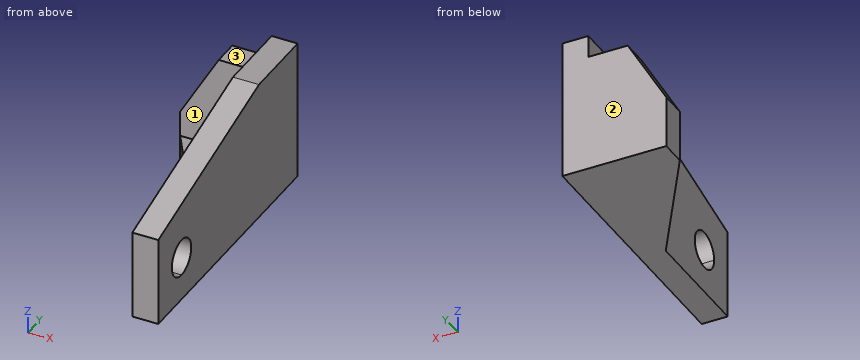
```python
from build123d import *

# Parameters (mm, degrees)
F0_W     = 33.3375
F0_H     = 11.1125
F0_W_2   = 11.1125
F1_DEPTH = 11.1125
F2_W     = 11.1125
F2_H     = 60.325
F3_DEPTH = 103.1875
F6_DEPTH = 25.4
F5_W     = 52.3875
F5_H     = 11.2454069465
F7_DEPTH = 33.3375
F9_DEPTH = 25.4


with BuildPart() as f1:
    # F0 (on Front) → F1 (new body)
    with BuildSketch(Plane.XZ):
        Polygon((-49.5353981066, -0.1329069465), (-16.1978981066, -0.1329069465), (-16.1978981066, 39.5545930535), (-33.0376141645, 39.5545930535), (-49.5353981066, 10.9795930535), align=None)
        with Locations((-32.8666481066, -5.6891569465)):
            Rectangle(F0_W, F0_H)
        with Locations((-10.6416481066, -5.6891569465)):
            Rectangle(F0_W_2, F0_H)
        Polygon((-16.1978981066, -0.1329069465), (-5.0853981066, -0.1329069465), (-5.0853981066, 49.0795930535), (-16.1978981066, 49.0795930535), (-16.1978981066, 39.5545930535), align=None)
    extrude(amount=F1_DEPTH)

    # F2 (on face) → F3 (join)
    with BuildSketch(Plane.XZ.offset(11.1125)):
        with Locations((-10.6416481066, 18.9170930535)):
            Rectangle(F2_W, F2_H)
    extrude(amount=F3_DEPTH)

    # F4 (on face) → F6 (cut)
    with BuildSketch(Plane(origin=(-16.1978981066, 0, 0), x_dir=(0, -1, 0), z_dir=(-1, 0, 0))):
        Polygon((114.3, 49.0795930535), (31.75, 49.0795930535), (114.3, 26.9603872183), align=None)
        with BuildLine():
            ThreePointArc((103.1875, 7.8045930535), (89.6373399243, 13.4172531291), (95.25, -0.1329069465))
            ThreePointArc((95.25, -0.1329069465), (100.8626600757, 2.1919329778), (103.1875, 7.8045930535))
        make_face()
    extrude(amount=-F6_DEPTH, mode=Mode.SUBTRACT)

    # F5 (on face) → F7 (join)
    with BuildSketch(Plane(origin=(-16.1978981066, 0, 0), x_dir=(0, -1, 0), z_dir=(-1, 0, 0))):
        with Locations((37.30625, -5.6227034733)):
            Rectangle(F5_W, F5_H)
    extrude(amount=F7_DEPTH)

    # F8 (on face) → F9 (cut)
    with BuildSketch(Plane.XY):
        Polygon((-16.1978981066, -63.5), (-49.5353981066, -11.1125), (-49.5353981066, -63.5), align=None)
    extrude(amount=-F9_DEPTH, mode=Mode.SUBTRACT)


solid = f1.part
```
Work out the finished part from the listing and answer in its coordinate system (mm). Face numbers are marked on the shaded views. A direction names the side the tool comes from. Give positions to 0.01 mm unless a question says otherwise; leave off trailing zeros. Order: outer loops, then holes, each group sorted by start corner. A loop starts at its lowest first (then second) coordinate and runs counter-clockwise, first axis right, second up.
1. Straight lines are drawn through the part: L1, parallel to Z at x = -27, y = -12; L2, parallel to X at y = -32, z = 11.5; L3, parallel to Y at x = -18.5, z = 32.5. For each, find the intervals that lie inside material, in ascending order.
Result sheet:
L1: z = -11.25 to 0
L2: x = -16.2 to -5.09
L3: y = -11.11 to 0
2. Section B-B, the plane y = -92.5 is taken. Determine the outline of the cut face in (x, z), and give its area (3 significant figures).
Result sheet:
outline: (-16.2, -11.25) - (-5.09, -11.25) - (-5.09, 0.36) - (-16.2, 0.36) - close; (-16.2, 15.25) - (-5.09, 15.25) - (-5.09, 32.8) - (-16.2, 32.8) - close
area: 324 mm2
3. For the marked faces 1, 2 and 3, determine the directions among +Z, -Z, +X, -X, +Y, -Y from which every point of the face is accessible in a straight line to the end or side of a thin tool.
Result sheet:
face 1: +Z, -X, -Y
face 2: +Z, -Z, +X, -X, +Y
face 3: +Z, -X, +Y, -Y
4. Section D-D, the plane y = -24 is taken. Determine the outline of the cut face in (x, z), and give its area (3 significant figures).
Result sheet:
outline: (-41.33, -11.25) - (-5.09, -11.25) - (-5.09, 49.08) - (-16.2, 49.08) - (-16.2, 0) - (-41.33, 0) - close
area: 953 mm2
5. Section C-C, the plane z = 36 is taken. Determine the outline of the cut face in (x, y), and give its area (3 significant figures).
Result sheet:
outline: (-35.09, -11.11) - (-16.2, -11.11) - (-16.2, -80.56) - (-5.09, -80.56) - (-5.09, 0) - (-35.09, 0) - close
area: 1,110 mm2
6. Each of these flat-tipped pins is pushed along its axis until it touches: P1, Ø1.5, axis at x = -26.5, z = 11, coming from the -Y side; P2, Ø10, axis at y = -80, z = 35.5, coming from the -X side; P3, Ø4, axis at y = -32, z = -3.5, coming from the -X side. Where does it stop, or does it pass through?
Result sheet:
P1: stops at y = -11.11
P2: stops at x = -16.2
P3: stops at x = -37.52
